CAD build for the part. Positions are in the model's coordinates, mm. Face numbers are marked on the shaded views. A direction names the side the tool comes from. Round coordinates to 2 decimals unless told otherwise and drop trailing zeros. Write each loop counter-clockwise with the first axis right and the second up, starting at its lowest first coordinate (ties: lowest second). Pieces come first, ordered by that corner, then holes. Notation, with made-up numbers: (48, -16) -> (105, -16) arc R37 cw to (105, 23) -> close; hole circle Ø7 at (54, 34.5). An arc over 180 degrees is marked (long way). Put each result on its own line as item: value. Start each with the question number.
1. Flat gauge pin, fed straight in: P1, Ø10, axis at x = 35.5, z = -21.5, coming from the +Y side. Where does the tip first touch, or does it go through?
2. Saw through at D-D on x = 63.5. List the corners of the cut face in (y, z), and give its area (3 significant figures).
3. Drill centre lines: line 1 (X direction, y = 7, z = -91); line 2 (Z direction, x = 6.5, y = 23.75); line 3 (X direction, y = 18.75, z = -83). Where is each one in solid material? Low to high. Write a range as from..to.
4. Saw through at B-B on z = -88. List the corners of the cut face in (x, y), and give its area (3 significant figures).
5. Saw through at C-C on x = 54.5. List the corners of the cut face in (y, z).
6. Pull direction X, two halves, no side cores. Call the marked faces 3, 4 and 5: pulls with the +X half, pulls with the -X half, needs draft (parallel to the pull), parting line crosses it, or undercut.
7. 3-axis set-ups, long thin cutter, end or side, ignore diameter. For the marked faces 1 and 2: which of +Z, -Z, +X, -X, +Y, -Y reach the whole face in a straight line?
8. Saw through at A-A on y = 5. List the corners of the cut face in (x, z).
from build123d import *

# Parameters (mm, degrees)
SKETCH1_W          = 66.04
SKETCH1_H          = 101.6
BASE_EXTRUDE_DEPTH = 2.54
SKETCH2_W          = 73.66
SKETCH2_H          = 109.22
SKETCH2_W_2        = 66.04
SKETCH2_H_2        = 101.6
WALLS_DEPTH        = 25.4
BUTTON_GUIDE_DEPTH = 22.86


with BuildPart() as part:
    # Sketch1 → Base Extrude (new body)
    with BuildSketch(Plane(origin=(0, 0, 0), x_dir=(1, 0, 0), z_dir=(0, 1, 0))):
        with Locations((33.02, 50.8)):
            Rectangle(SKETCH1_W, SKETCH1_H)
    extrude(amount=BASE_EXTRUDE_DEPTH)

    # Sketch2 → Walls (add)
    with BuildSketch(Plane.XZ):
        with Locations((33.02, -50.8)):
            Rectangle(SKETCH2_W, SKETCH2_H)
        with Locations((33.02, -50.8)):
            Rectangle(SKETCH2_W_2, SKETCH2_H_2, mode=Mode.SUBTRACT)
    extrude(amount=-WALLS_DEPTH)

    # Sketch3 → Button Guide (add)
    with BuildSketch(Plane(origin=(0, 25.4, 0), x_dir=(1, 0, 0), z_dir=(0, 1, 0))):
        Polygon((3.81, 86.36), (0, 84.583367822), (0, 76.2), (3.81, 76.2), align=None)
        Polygon((28.703367822, 101.6), (0, 101.6), (0, 93.216632178), (3.81, 91.44), (3.81, 97.79), (30.48, 97.79), align=None)
        Polygon((66.04, 101.6), (37.336632178, 101.6), (35.56, 97.79), (62.23, 97.79), (62.23, 91.44), (66.04, 93.216632178), align=None)
        Polygon((66.04, 76.2), (66.04, 84.583367822), (62.23, 86.36), (62.23, 76.2), align=None)
    extrude(amount=-BUTTON_GUIDE_DEPTH)


solid = part.part
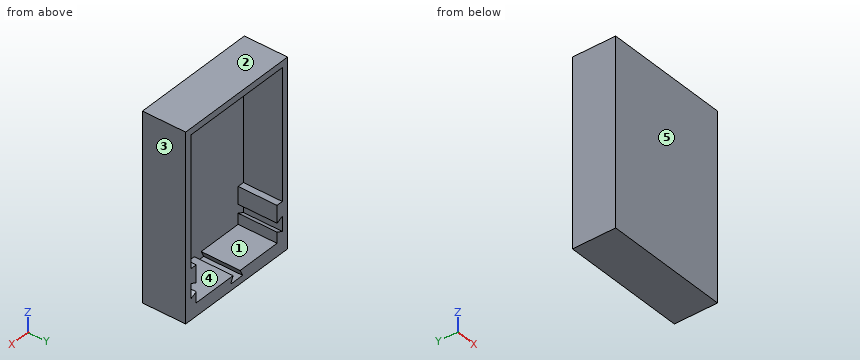
Return value:
1. P1: stops at y = 2.54
2. outline: (0, -105.41) -> (25.4, -105.41) -> (25.4, -92.03) -> (2.54, -92.03) -> (2.54, -85.77) -> (25.4, -85.77) -> (25.4, -76.2) -> (2.54, -76.2) -> (2.54, 0) -> (25.4, 0) -> (25.4, 3.81) -> (0, 3.81) -> close
2. area: 889 mm^2
3. line 1: x = -3.81..0, 66.04..69.85
3. line 2: z = -105.41..-97.79, 0..3.81
3. line 3: x = -3.81..3.81, 62.23..69.85
4. outline: (-3.81, 0) -> (69.85, 0) -> (69.85, 25.4) -> (66.04, 25.4) -> (66.04, 2.54) -> (0, 2.54) -> (0, 25.4) -> (-3.81, 25.4) -> close
4. area: 361 mm^2
5. outline: (0, -105.41) -> (25.4, -105.41) -> (25.4, -97.79) -> (2.54, -97.79) -> (2.54, 0) -> (25.4, 0) -> (25.4, 3.81) -> (0, 3.81) -> close
6. face 3: pulls with the +X half
6. face 4: undercut
6. face 5: needs draft
7. face 1: +Y
7. face 2: +Z, +X, -X, +Y, -Y
8. outline: (-3.81, -105.41) -> (69.85, -105.41) -> (69.85, 3.81) -> (-3.81, 3.81) -> close; hole (0, -93.22) -> (3.81, -91.44) -> (3.81, -97.79) -> (30.48, -97.79) -> (28.7, -101.6) -> (37.34, -101.6) -> (35.56, -97.79) -> (62.23, -97.79) -> (62.23, -91.44) -> (66.04, -93.22) -> (66.04, -84.58) -> (62.23, -86.36) -> (62.23, -76.2) -> (66.04, -76.2) -> (66.04, 0) -> (0, 0) -> (0, -76.2) -> (3.81, -76.2) -> (3.81, -86.36) -> (0, -84.58) -> close
